Design review of the part built by this model. Coordinates are the model's own, in mm. Face numbers are marked on the shaded views. A direction names the side the tool comes from. Give positions to 0.01 mm unless a question says otherwise; leave off trailing zeros. Write each loop counter-clockwise with the first axis right and the second up, starting at its lowest first coordinate (ties: lowest second). Pieces come first, ordered by that corner, then holes.
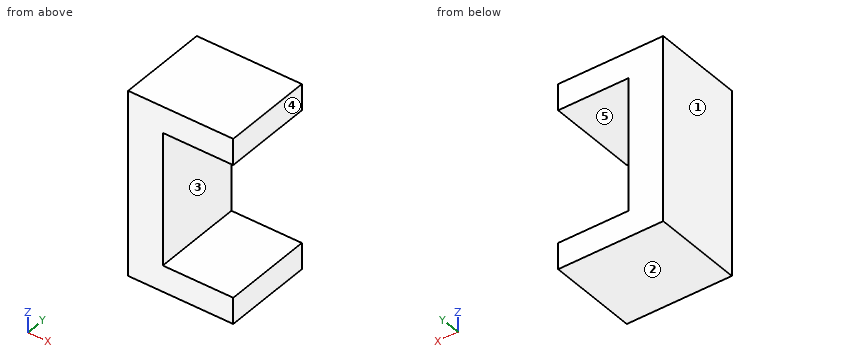
Autodesk Inventor part; units mm, degrees
ref_plane "YZ Plane" through (0, 0, 0) normal (1, 0, 0) x (0, 1, 0)
ref_plane "XZ Plane" through (0, 0, 0) normal (0, 1, 0) x (-1, 0, 0)
ref_plane "XY Plane" through (0, 0, 0) normal (0, 0, 1) x (1, 0, 0)
sketch "Sketch1" plane through (0, 0, 0) normal (0, 1, 0) x (-1, 0, 0)
  line L0 (0, -11.5) -> (0, 11.5) construction
  line L1 (0, -16.05) -> (0, 16.05) construction
  line L2 (0, -16.05) -> (-12.2, -16.05)
  line L3 (-12.2, -16.05) -> (-12.2, -11.5)
  line L4 (-12.2, -11.5) -> (0, -11.5)
  line L5 (0, -11.5) -> (0, -16.05) construction
  line L6 (0, 11.5) -> (-12.2, 11.5)
  line L7 (-12.2, 11.5) -> (-12.2, 16.05)
  line L8 (-12.2, 16.05) -> (0, 16.05)
  line L9 (0, 16.05) -> (0, 11.5) construction
  line L10 (0, -16.05) -> (6, -16.05)
  line L11 (6, -16.05) -> (6, 16.05)
  line L12 (6, 16.05) -> (0, 16.05)
  line L13 (0, -11.5) -> (0, 11.5)
  point P0 (0, 0)
  point P1 (0, 0)
  dimension "d0" = 23
  dimension "d1" = 32.1
  dimension "d2" = 12.2
  dimension "d3" = 6
extrude "Extrusion1" add sketch "Sketch1" along normal blind 15.7
sketch "Sketch2" plane through (12.2, 0, -16.05) normal (0, 0, -1) x (-1, 0, 0)
  line L0 (18.2, 0) -> (18.2, 15.7)
  line L1 (18.2, 9.2581) -> (21.2, 10.35)
  line L2 (21.2, 10.35) -> (21.2, 5.35)
  line L3 (21.2, 5.35) -> (18.2, 6.4419)
  line L4 (18.2, 7.85) -> (21.2, 7.85) construction
  point P0 (12.2, 0)
  dimension "d6" = 3
  dimension "d7" = 70
  dimension "d8" = 5
properties part number "Soporte Servo SG90"
(1) Consider section C-C, the plane z = 6. Give the boundary of the cut face in (x, y), then the cut area to 3 significant figures.
Resolved:
outline: (-6, 0) - (0, 0) - (0, 15.7) - (-6, 15.7) - close
area: 94.2 mm2
(2) To check wall thickness, follow L1, parallel to Z at x = 9.25, y = 10.25; L2, parallel to X at y = 7.25, z = 8. State the ranges of each line that lie inside material, in increasing order.
Resolved:
L1: z = -16.05 to -11.5, 11.5 to 16.05
L2: x = -6 to 0
(3) Tool access review of the marked faces 4 and 5: name each direction out of +Z, -Z, +X, -X, +Y, -Y from which nothing blocks a thin tool from reaching the whole face with its end or side.
Resolved:
face 4: +Z, -Z, +X, +Y, -Y
face 5: +X, +Y, -Y
(4) Consider section A-A, the plane x = 6.25. Give the boundary of the cut face in (y, z).
Resolved:
outline: (0, -16.05) - (15.7, -16.05) - (15.7, -11.5) - (0, -11.5) - close; (0, 11.5) - (15.7, 11.5) - (15.7, 16.05) - (0, 16.05) - close
(5) Consider section B-B, the plane y = 5.25. Give the boundary of the cut face in (x, z).
Resolved:
outline: (-6, -16.05) - (12.2, -16.05) - (12.2, -11.5) - (0, -11.5) - (0, 11.5) - (12.2, 11.5) - (12.2, 16.05) - (-6, 16.05) - close
(6) Mouldability with a two-part tool opening along Z and no side actions: class the marked faces 1, 2 and 3 as pulls with the +Z half, pulls with the -Z half, needs draft (parallel to the pull), parting line crosses it, or undercut.
Resolved:
face 1: needs draft
face 2: pulls with the -Z half
face 3: undercut
(7) Clearance check with a flat-ended pin moving along its axis: P1, Ø1.5, axis at y = 9, z = -1.5, coming from the +X side. State where the tip first meets the part, or that it passes through.
Resolved:
P1: stops at x = 0
